The drawing under review shows one solid part. Ordinate dimensions are in mm from its lowest x, y, z. Coordinates: 2 decimals unless noted, no trailing zeros. Write each loop counter-clockwise with the first axis right and the second up, starting at its lowest first coordinate (ties: lowest second). Pieces come first, ordered by that corner, then holes.
Q1. Take a section at D-D (z = 10.75). Give the boundary of the cut face in (x, y).
Q2. For probe 1 along Y at (x, z) = (6, 13.6); probe 2 along Z at (x, y) = (2.75, 10.25); probe 3 along Y at (x, z) = (11.25, 10.5), list the stretches that pass through material, from the lowest coordinate up.
Q3. Take a section at C-C (x = 9.75). Give the boundary of the cut face in (y, z).
Q4. Mouldability with a two-part tool opening along Y and no side actions: class the marked faces 1, 2 and 3 as pulls with the +Y half, pulls with the -Y half, needs draft (parallel to the pull), parting line crosses it, or undercut.
Q5. Insertion check: pin 1 (2 mm diameter, centred on y = 6, z = 5.5, fed in from +X); pin 2 (3 mm diameter, centred on x = 6, y = 6, fed in from -Z); pin 3 (6 mm diameter, centred on x = 8, y = 3.5, fed in from -Z). Each pin has a flat end and moves straight along its axis. Give the tip position at first contact, or say it passes through.
Q6. Take a section at A-A (y = 6). Give the boundary of the cut face in (x, z), and give its area (3 significant figures).
Q7. Take a section at B-B (z = 4.25). Give the boundary of the cut face in (x, y).
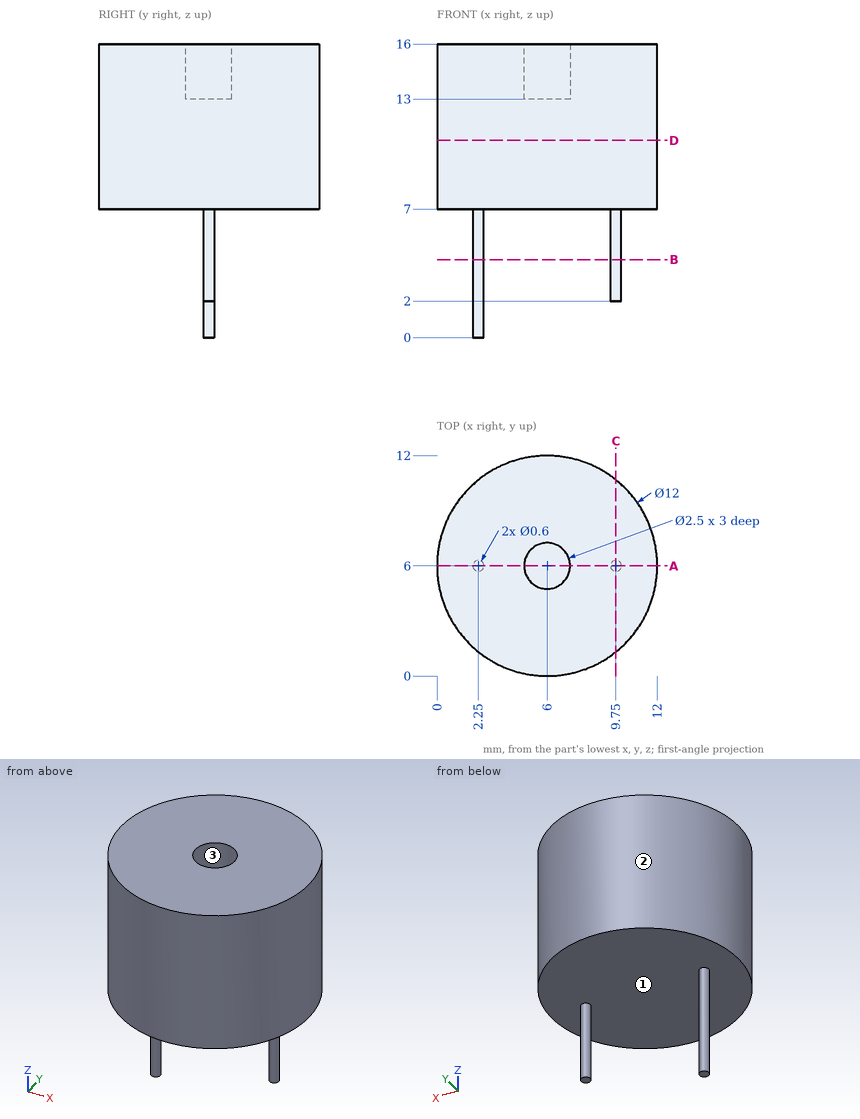
Response:
1. outline: circle Ø12 at (6, 6)
2. probe 1: y = 0 to 4.75, 7.25 to 12
2. probe 2: z = 7 to 16
2. probe 3: y = 3.1 to 8.9
3. outline: (1.32, 7) - (5.7, 7) - (5.7, 2) - (6.3, 2) - (6.3, 7) - (10.68, 7) - (10.68, 16) - (1.32, 16) - close
4. face 1: needs draft
4. face 2: parting line crosses it
4. face 3: undercut
5. pin 1: stops at x = 10.05
5. pin 2: stops at z = 7
5. pin 3: stops at z = 2
6. outline: (0, 7) - (1.95, 7) - (1.95, 0) - (2.55, 0) - (2.55, 7) - (9.45, 7) - (9.45, 2) - (10.05, 2) - (10.05, 7) - (12, 7) - (12, 16) - (7.25, 16) - (7.25, 13) - (4.75, 13) - (4.75, 16) - (0, 16) - close
6. area: 108 mm2
7. outline: circle Ø0.6 at (2.25, 6); circle Ø0.6 at (9.75, 6)
